from build123d import *

# Parameters (mm, degrees)
F0_W           = 130
F0_H           = 180
F1_DEPTH       = 9
F3_D           = 5
F3_DEPTH       = 15
F3_CBORE_D     = 6
F3_CBORE_DEPTH = 3
F3_TIP         = 1.5021515476
F4_SIZE        = 5


with BuildPart() as f1:
    # F0 (on Top) → F1 (new body, symmetric)
    with BuildSketch(Plane.XY):
        Rectangle(F0_W, F0_H)
    extrude(amount=F1_DEPTH, both=True)

    # F3
    with Locations(Plane.XY.offset(9)):
        with Locations((-56, 65), (56, 65), (56, -65), (-56, -65)):
            CounterBoreHole(F3_D / 2, F3_CBORE_D / 2, F3_CBORE_DEPTH, depth=F3_DEPTH)
            with Locations((0, 0, -(F3_DEPTH + F3_TIP / 2))):  # 118° drill point
                Cone(0, F3_D / 2, F3_TIP, mode=Mode.SUBTRACT)

    # F4
    f4_edges = [f1.edges().sort_by_distance(p)[0] for p in [
        (-65, 0, 9),
        (65, 0, 9),
    ]]
    chamfer(f4_edges, length=F4_SIZE)


solid = f1.part
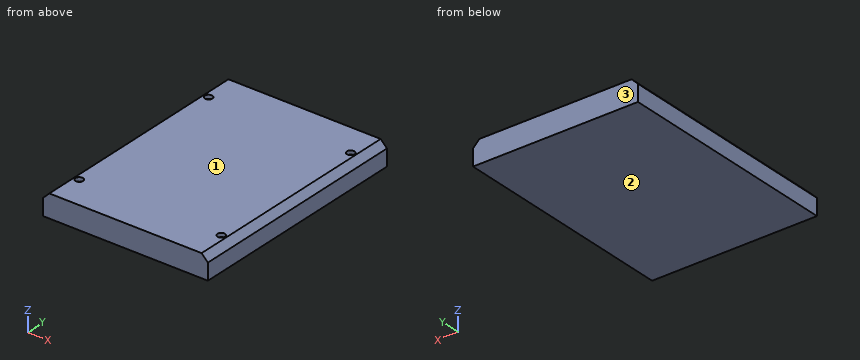
Geometry check sheet. Reference: the model listing, model coordinates, mm. Face numbers are marked on the shaded views. Give positions to 0.01 mm unless a question says otherwise; leave off trailing zeros. Answer as a JSON object with one key per item and string values.
(1) Depth check by flat-ended pin: pin 1 Ø3 at (x, y) = (56, 65) entering from +Z; pin 2 Ø1 at (y, z) = (54.5, 5.5) entering from +X; pin 3 Ø5.5 at (x, y) = (56, 65) entering from +Z. Enter the tip coordinate at first touch or a pass-through.
Report:
{"pin 1": "z = -6.6", "pin 2": "x = 64", "pin 3": "z = 6"}
(2) Material ranges on line 1 (Y direction, x = -56, z = -2); line 2 (Y direction, x = 56, z = 8.3); line 3 (X direction, y = -65, z = 3.25), recorded low to high.
Report:
{"line 1": "-90 to -67.5, -62.5 to 62.5, 67.5 to 90", "line 2": "-90 to -68, -62 to 62, 68 to 90", "line 3": "-65 to -58.5, -53.5 to 53.5, 58.5 to 65"}
(3) Draft check along Z on the marked faces 1, 2 and 3. Enter one of: released by +Z, released by -Z, zero draft, split by the parting line, or undercut.
Report:
{"face 1": "released by +Z", "face 2": "released by -Z", "face 3": "zero draft"}
